```python
from build123d import *

# Parameters (mm, degrees)
BOSS_EXTRUDE1_DEPTH = 10
CUT_EXTRUDE1_DEPTH  = 5.1
SKETCH2_R           = 1.7
CUT_EXTRUDE2_DEPTH  = 5.1


with BuildPart() as part:
    # Sketch1 → Boss-Extrude1 (new body)
    with BuildSketch(Plane.XY):
        Polygon((-27.22, 20), (-10, -135.135135135), (10, -135.135135135), (27.22, 20), align=None)
    extrude(amount=BOSS_EXTRUDE1_DEPTH)

    # Sketch1_3 → Cut-Extrude1 (cut)
    with BuildSketch(Plane.XY):
        Polygon((-25, 0), (25, 0), (27.22, 20), (-27.22, 20), align=None)
    extrude(amount=CUT_EXTRUDE1_DEPTH, mode=Mode.SUBTRACT)

    # Sketch2 → Cut-Extrude2 (cut)
    with BuildSketch(Plane(origin=(0, 0, 5.1), x_dir=(-1, 0, 0), z_dir=(0, 0, -1))):
        with Locations((-15, 10)):
            Circle(SKETCH2_R)
        with Locations((15, 10)):
            Circle(SKETCH2_R)
    extrude(amount=-CUT_EXTRUDE2_DEPTH, mode=Mode.SUBTRACT)


solid = part.part
```
Source: CAD feature listing. Evaluate the final solid. Frame: model axes, mm. A direction names the side the tool comes from. Round coordinates to 2 decimals unless told otherwise and drop trailing zeros. Write each loop counter-clockwise with the first axis right and the second up, starting at its lowest first coordinate (ties: lowest second). Pieces come first, ordered by that corner, then holes. Notation, with made-up numbers: M -38.5,-11.75 L -28.5,-11.75 A25 ccw -28.5,21.25 Z; hole C 24.25,69 d11. An arc over 180 degrees is marked long. Use CSV: the item, a comma, the result in double quotes. Start each with the question number.
Q1. Pull-direction query (X, two-part tool) for faces 1 (the face through (18.49, -58.65, 4.93)), 2 (the face through (0, 10, 5.1)), 3 (the face through (-16.57, 9.35, 7.52)); classes: +X half, -X half, draft (parallel to the pull), parting line (faces both ways), or undercut.
Q2. First-contact query: P1, Ø5.5, axis at x = 7.5, z = 2, coming from the +Y side; P2, Ø4, axis at y = -106, z = 4, coming from the -X side. Flat tips, straight axial feed; report the tip coordinate or a pass-through.
Q3. Cut plane B-B on x = 2. Output: boundary loops of the cut face in (y, z), plus the area to 3 significant figures.
Q4. Cut plane A-A on y = 10. Output: boundary loops of the cut face in (x, z).
Q5. Cut plane D-D on x = -15. Output: boundary loops of the cut face in (y, z), plus the area to 3 significant figures.
Q6. Cut plane C-C on z = 8.5. Output: boundary loops of the cut face in (x, y).
Q7. Access query for faces 4 (the face through (13.43, 9.35, 7.52)), 5 (the face through (0, 0, 3)). Directions: +Z, -Z, +X, -X, +Y, -Y. A direction counts if a zero-diameter tool reaches every point of the face in a straight line with its end or side. Return the directions, or none.
Q8. Line query: line 1 (X direction, y = -42, z = 9.75); line 2 (X direction, y = -12.5, z = 0.5); line 3 (Y direction, x = -7, z = 4). Output: solid intervals per line, ascending. Write a range as from..to.
Results found:
1,face 1,"+X half"
1,face 2,"draft"
1,face 3,"undercut"
2,P1,"y = 0"
2,P2,"x = -13.46"
3,outline,"M -135.14,0 L 0,0 L 0,5.1 L 20,5.1 L 20,10 L -135.14,10 Z"
3,area,"1,450 mm^2"
4,outline,"M -26.11,5.1 L -16.7,5.1 L -16.7,10 L -26.11,10 Z; M -13.3,5.1 L 13.3,5.1 L 13.3,10 L -13.3,10 Z; M 16.7,5.1 L 26.11,5.1 L 26.11,10 L 16.7,10 Z"
5,outline,"M -90.09,0 L 0,0 L 0,5.1 L 8.3,5.1 L 8.3,10 L -90.09,10 Z; M 11.7,5.1 L 20,5.1 L 20,10 L 11.7,10 Z"
5,area,"982 mm^2"
6,outline,"M -27.22,20 L -10,-135.14 L 10,-135.14 L 27.22,20 Z; hole C -15,10 d3.4; hole C 15,10 d3.4"
7,face 4,"+Z, -Z"
7,face 5,"-Z, +X, -X, +Y"
8,line 1,"-20.34..20.34"
8,line 2,"-23.61..23.61"
8,line 3,"-135.14..0"
